Geometry: final body of the model. Coordinates: model frame, mm. Face numbers are marked on the shaded views. A direction names the side the tool comes from. Give positions to 0.01 mm unless a question says otherwise; leave off trailing zeros. Loops run counter-clockwise (first coordinate to the right, second up) from the corner with the lowest first, then second, coordinate; pieces in that order, holes last.
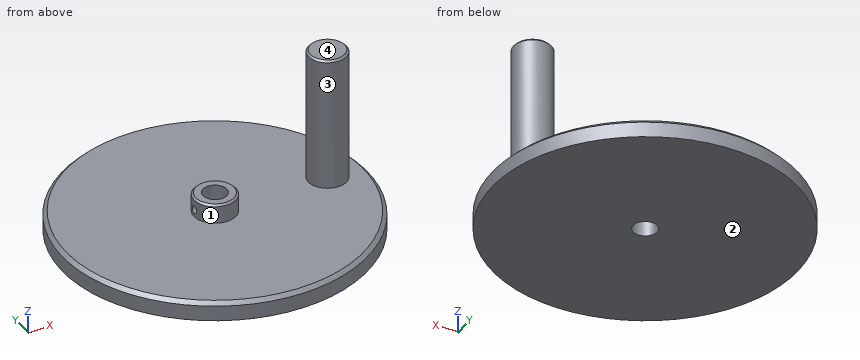
from build123d import *

# Parameters (mm, degrees)
F0_R     = 50.8
F0_R_2   = 7
F0_R_3   = 6.35
F1_DEPTH = 6.35
F2_DEPTH = 50.8
F0_R_4   = 4
F3_DEPTH = 12.7
F4_SIZE  = 0.635
F5_R     = 1.25
F6_DEPTH = 25.4
F7_SIZE  = 1.27


with BuildPart() as f1:
    # F0 (on Top) → F1 (new body)
    with BuildSketch(Plane.XY):
        Circle(F0_R)
        Circle(F0_R_2, mode=Mode.SUBTRACT)
        with Locations((38.1, 0)):
            Circle(F0_R_3, mode=Mode.SUBTRACT)
    extrude(amount=F1_DEPTH)

    # F0 (on Top) → F2 (join)
    with BuildSketch(Plane.XY):
        with Locations((38.1, 0)):
            Circle(F0_R_3)
    extrude(amount=F2_DEPTH)

    # F0 (on Top) → F3 (join)
    with BuildSketch(Plane.XY):
        Circle(F0_R_2)
        Circle(F0_R_4, mode=Mode.SUBTRACT)
    extrude(amount=F3_DEPTH)

    # F4
    f4_edges = [f1.edges().sort_by_distance(p)[0] for p in [
        (31.75, 0, 50.8),
        (-7, 0, 12.7),
    ]]
    chamfer(f4_edges, length=F4_SIZE)

    # F5 (on Right) → F6 (cut)
    with BuildSketch(Plane.YZ):
        with Locations((0, 8.89)):
            Circle(F5_R)
    extrude(amount=-F6_DEPTH, mode=Mode.SUBTRACT)

    # F7
    f7_edges = [f1.edges().sort_by_distance(p)[0] for p in [
        (-50.8, 0, 6.35),
    ]]
    chamfer(f7_edges, length=F7_SIZE)


solid = f1.part
Item 1: Ray query, probe 1 along Y at (x, z) = (0, 10); probe 2 along Z at (x, y) = (43, 7.5); probe 3 along Y at (x, z) = (0, 3). Return the intervals inside material, ascending.
Values follow:
probe 1: y = -7 to -4, 4 to 7
probe 2: z = 0 to 6.35
probe 3: y = -50.8 to -4, 4 to 50.8
Item 2: Section query A-A on x = 0. Return loops of the section in (y, z) (3 decimals), plus the area to 3 significant figures.
Values follow:
outline: (-50.8, 0) - (-4, 0) - (-4, 12.7) - (-6.365, 12.7) - (-7, 12.065) - (-7, 6.35) - (-49.53, 6.35) - (-50.8, 5.08) - close; (4, 0) - (50.8, 0) - (50.8, 5.08) - (49.53, 6.35) - (7, 6.35) - (7, 12.065) - (6.365, 12.7) - (4, 12.7) - close
area: 630 mm2
Item 3: Section query B-B on y = 0. Return loops of the section in (x, z) (3 decimals).
Values follow:
outline: (-50.8, 0) - (-4, 0) - (-4, 7.64) - (-7, 7.64) - (-7, 6.35) - (-49.53, 6.35) - (-50.8, 5.08) - close; (-7, 10.14) - (-4, 10.14) - (-4, 12.7) - (-6.365, 12.7) - (-7, 12.065) - close; (4, 0) - (50.8, 0) - (50.8, 5.08) - (49.53, 6.35) - (44.45, 6.35) - (44.45, 50.165) - (43.815, 50.8) - (32.385, 50.8) - (31.75, 50.165) - (31.75, 6.35) - (7, 6.35) - (7, 12.065) - (6.365, 12.7) - (4, 12.7) - close
Item 4: Set-up query: the marked faces 3 and 4. Return all of +Z, -Z, +X, -X, +Y, -Y with unobstructed straight access to the full face (end or side cutting, diameter ignored); none if empty.
Values follow:
face 3: +Z
face 4: +Z, +X, -X, +Y, -Y
Item 5: Pin query (flat end, axial travel): pin 1 (1 mm diameter, centred on x = 28.5, y = -10, fed in from +Z); pin 2 (10 mm diameter, centred on y = -12, z = 9, fed in from -X) (3 decimals); pin 3 (10 mm diameter, centred on x = -1.5, y = 2, fed in from +Z). Return the tip coordinate at first contact, or that it passes through.
Values follow:
pin 1: stops at z = 6.35
pin 2: stops at x = -50.015
pin 3: stops at z = 12.7
Item 6: Section query D-D on z = 33. Return loops of the section in (x, y).
Values follow:
outline: circle Ø12.7 at (38.1, 0)
Item 7: Section query C-C on z = 8.89. Return loops of the section in (x, y).
Values follow:
outline: (-6.89, -1.25) arc R7 ccw (long way) to (-6.89, 1.25) - (-3.8, 1.25) arc R4 cw (long way) to (-3.8, -1.25) - close; circle Ø12.7 at (38.1, 0)
Item 8: Draft query along X for the marked faces 1 and 2. Return one class per face: +X half, -X half, draft (parallel to the pull), parting line (faces both ways), or undercut.
Values follow:
face 1: undercut
face 2: draft
